Geometry: final body of the model. Coordinates: model frame, mm. Give positions to 0.01 mm unless a question says otherwise; leave off trailing zeros. Write each loop counter-clockwise with the first axis right and the second up, starting at its lowest first coordinate (ties: lowest second). Pieces come first, ordered by that corner, then holes. Notation, with made-up numbers: (2, 66.5) -> (48, 66.5) arc R13 ccw to (48, 86.5) -> close; hole circle Ø10 at (45, -4.75). An arc over 180 degrees is marked (long way). Answer as a JSON object with one key per item and string values. Group by question number.
(1) Contact query for flat-ended pins moving along their axis: pin 1 Ø1.5 at (y, z) = (-7, 9) entering from +X; pin 2 Ø3 at (x, z) = (-4.5, 14) entering from +Y; pin 3 Ø8 at (x, z) = (-5, 3) entering from -Y; pin 4 Ø3 at (x, y) = (0, 0) entering from -Z. Output: stop coordinate, or through.
(2) Section query A-A on x = 0. Output: boundary loops of the cut face in (y, z).
(3) Draft query along X for faces 1 (the face through (-14.985, 0.66, 9.86)), 2 (the face through (9.52, 5.51, 10.14)), 3 (the face through (4, 7, 5)). Return one class per face: +X half, -X half, draft (parallel to the pull), parting line (faces both ways), or undercut.
(4) Section query C-C on z = 9. State how many separate pieces and enclosed holes the cut face has, plus the area to 3 significant figures.
(5) Material intervals for probe 1 along Y at (x, z) = (0, 11.75); probe 2 along Y at (x, z) = (-9, 13.75); probe 3 along Y at (x, z) = (7.75, 7.25), sorted ascending.
(6) Section query B-B on y = 0. Output: boundary loops of the cut face in (x, z).
from build123d import *

# Parameters (mm, degrees)
SKETCH1_R               = 15
SKETCH1_R_2             = 2.5
BOSS_EXTRUDE1_DEPTH     = 20
SHELL1_T                = -5
SKETCH2_W               = 1
SKETCH2_H               = 3
CUT_EXTRUDE_THIN1_DEPTH = 30.154759474
CIRPATTERN1_COUNT       = 30


with BuildPart() as part:
    # Sketch1 → Boss-Extrude1 (new body)
    with BuildSketch(Plane.XY):
        Circle(SKETCH1_R)
        Circle(SKETCH1_R_2, mode=Mode.SUBTRACT)
    extrude(amount=BOSS_EXTRUDE1_DEPTH)

    # Shell1
    shell1_openings = [part.faces().sort_by_distance(p)[0] for p in [
        (-14.575735931, 0, 20),
    ]]
    offset(amount=SHELL1_T, openings=shell1_openings, kind=Kind.INTERSECTION)

    # Sketch2 → Cut-Extrude-Thin1 (cut, symmetric)
    with BuildSketch(Plane.XY):
        with Locations((0, 12.5)):
            Rectangle(SKETCH2_W, SKETCH2_H)
    cut_extrude_thin1 = extrude(amount=CUT_EXTRUDE_THIN1_DEPTH, both=True, mode=Mode.SUBTRACT)

    # CirPattern1: Cut-Extrude-Thin1 ×30 about axis
    cirpattern1_axis = Axis((0, 0, 0), (0, 0, 1))
    for i in range(1, CIRPATTERN1_COUNT):
        add(cut_extrude_thin1.rotate(cirpattern1_axis, i * 360 / CIRPATTERN1_COUNT), mode=Mode.SUBTRACT)


solid = part.part
Answer list:
{
 "1": {"pin 1": "x = 13.64", "pin 2": "y = 14.7", "pin 3": "y = -14.97", "pin 4": "through"},
 "2": {"outline": "(-15, 0) -> (-14, 0) -> (-14, 20) -> (-15, 20) -> close; (-11, 0) -> (-2.5, 0) -> (-2.5, 20) -> (-7.5, 20) -> (-7.5, 5) -> (-10, 5) -> (-10, 20) -> (-11, 20) -> close; (2.5, 0) -> (11, 0) -> (11, 20) -> (10, 20) -> (10, 5) -> (7.5, 5) -> (7.5, 20) -> (2.5, 20) -> close; (14, 0) -> (15, 0) -> (15, 20) -> (14, 20) -> close"},
 "3": {"face 1": "parting line", "face 2": "undercut", "face 3": "undercut"},
 "4": {"separate pieces": "2", "enclosed holes": "32", "area": "460 mm2"},
 "5": {"probe 1": "-15 to -14, -11 to -10, -7.5 to -2.5, 2.5 to 7.5, 10 to 11, 14 to 15", "probe 2": "-12 to -8.78, -7.43 to -4.36, 4.36 to 7.43, 8.78 to 12", "probe 3": "-12.84 to -11.52, -9.82 to -6.32, 6.32 to 9.82, 11.52 to 12.84"},
 "6": {"outline": "(-15, 0) -> (-2.5, 0) -> (-2.5, 20) -> (-7.5, 20) -> (-7.5, 5) -> (-10, 5) -> (-10, 20) -> (-15, 20) -> close; (2.5, 0) -> (15, 0) -> (15, 20) -> (10, 20) -> (10, 5) -> (7.5, 5) -> (7.5, 20) -> (2.5, 20) -> close"}
}
